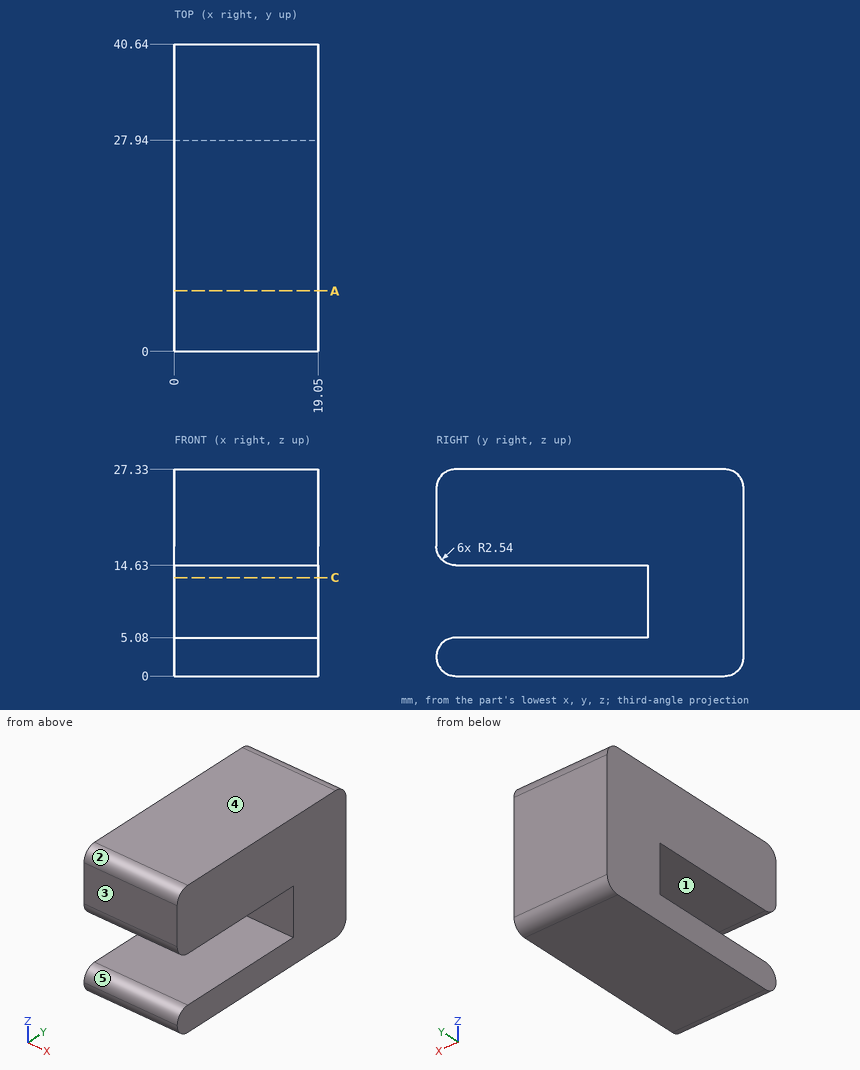
The figure shows three views and two pictorial views of one solid part (mm, origin at its lowest corner). Answer the questions. A direction names the side the tool comes from. Coordinates: 2 decimals unless noted, no trailing zeros. Write each loop counter-clockwise with the first axis right and the second up, starting at its lowest first coordinate (ties: lowest second). Pieces come first, ordered by that corner, then holes. Notation, with made-up numbers: (12.5, -12.75) -> (62.5, -12.75) arc R22 ccw to (62.5, 13.25) -> close; hole circle Ø10 at (70, 9.25). An arc over 180 degrees is marked (long way). Return JSON: item names as keys, results as strings.
1. A tool of negligible diameter and unlimited length cuts with its end or side. For the marked faces 4 and 5, from which of +Z, -Z, +X, -X, +Y, -Y can it reach the whole face along a straight path? Write none if from no direction.
Found:
{"face 4": "+Z, +X, -X, +Y, -Y", "face 5": "+X, -X, -Y"}
2. A cutting plane is placed at C-C (z = 13). Determine the outline of the cut face in (x, y), and give its area (3 significant figures).
Found:
{"outline": "(0, 27.94) -> (19.05, 27.94) -> (19.05, 40.64) -> (0, 40.64) -> close", "area": "242 mm2"}
3. Determine the mould class of the marked faces 1, 2 and 3 for opening direction Z: pulls with the +Z half, pulls with the -Z half, needs draft (parallel to the pull), parting line crosses it, or undercut.
Found:
{"face 1": "undercut", "face 2": "pulls with the +Z half", "face 3": "needs draft"}
4. Each of these flat-tipped pins is pushed along its axis until it touches: P1, Ø1.5, axis at y = 23, z = 14.5, coming from the +X side; P2, Ø3, axis at x = 14, z = 11, coming from the -Y side. Where does it stop, or does it pass through?
Found:
{"P1": "x = 19.05", "P2": "y = 27.94"}
5. A cutting plane is placed at A-A (y = 8). Determine the outline of the cut face in (x, z).
Found:
{"outline": "(0, 0) -> (19.05, 0) -> (19.05, 5.08) -> (0, 5.08) -> close; (0, 14.63) -> (19.05, 14.63) -> (19.05, 27.33) -> (0, 27.33) -> close"}
6. Find the intervals of material crossed by line 1 along Z through (x, y) = (8.75, 5); line 2 along Y through (x, z) = (1, 10); line 3 along Y through (x, z) = (8.5, 17) (1 decimal), in increasing order. Write a range as from..to.
Found:
{"line 1": "0..5.08, 14.63..27.33", "line 2": "27.94..40.64", "line 3": "0..40.6"}
